Verification items for this drawing (mm, ordinates from the low corner). A direction names the side the tool comes from. Coordinates: 2 decimals unless noted, no trailing zeros. Loops run counter-clockwise (first coordinate to the right, second up) from the corner with the lowest first, then second, coordinate; pieces in that order, holes last. Notation, with made-up numbers: (31, -29) -> (57, -29) arc R15 ccw to (57, -13) -> close; hole circle Ø3 at (47, -5.5). An arc over 180 degrees is marked (long way). Write item = value, one per line.
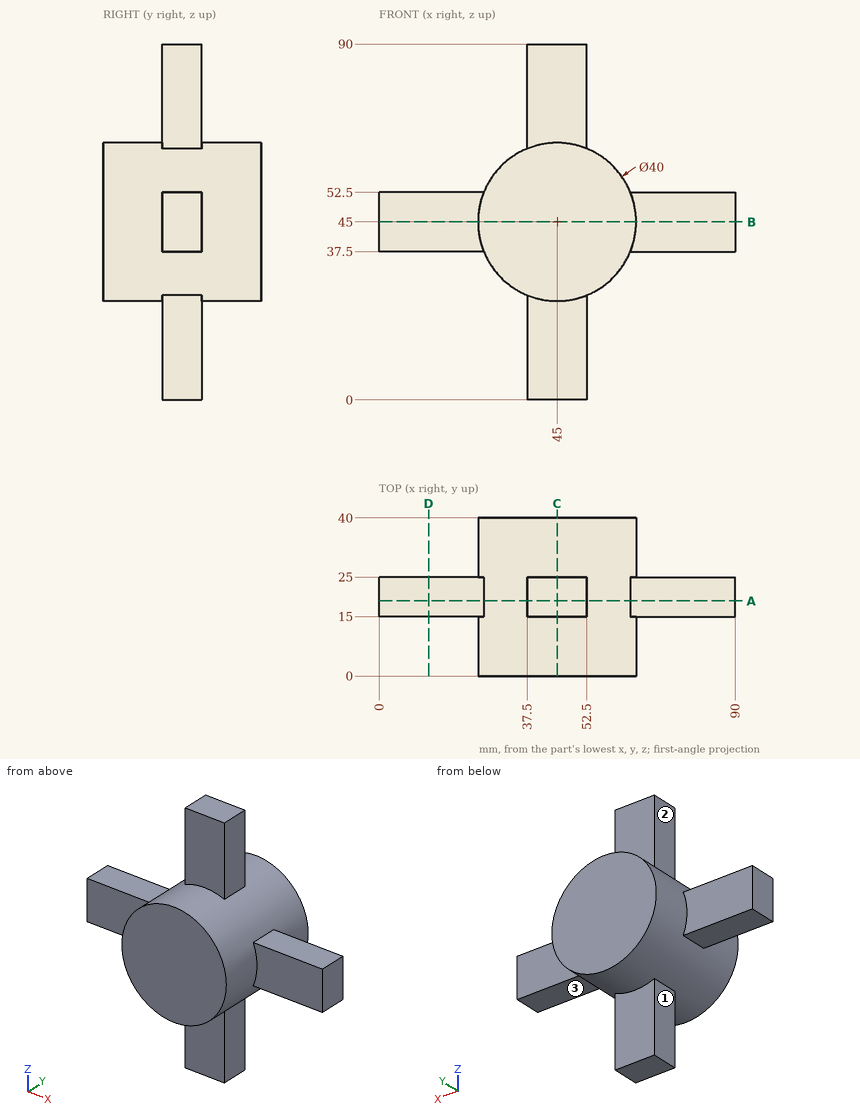
1) Tool access check on the marked faces 1, 2 and 3. Record the directions out of +Z, -Z, +X, -X, +Y, -Y that give a thin tool (end or side, any length) a straight path to the whole face; none if there is none.
Ans:
face_1 = -Z, -X, +Y, -Y
face_2 = +Z, -X, +Y, -Y
face_3 = -Z, +X, +Y, -Y
2) Depth check by flat-ended pin: pin 1 Ø8 at (x, z) = (52, 19) entering from +Y; pin 2 Ø2 at (x, y) = (48, 31.5) entering from -Z; pin 3 Ø11 at (y, z) = (17.5, 73) entering from +X. Enter the tip coordinate at first touch or a pass-through.
Ans:
pin_1 = 25
pin_2 = 25.1
pin_3 = 52.5
3) Sectioned sample at B-B, the plane z = 45. Record the cut outline in (x, y).
Ans:
outline = (0, 15) -> (25, 15) -> (25, 0) -> (65, 0) -> (65, 15) -> (90, 15) -> (90, 25) -> (65, 25) -> (65, 40) -> (25, 40) -> (25, 25) -> (0, 25) -> close
4) Sectioned sample at A-A, the plane y = 19. Record the cut outline in (x, z).
Ans:
outline = (0, 37.5) -> (26.46, 37.5) arc R20 ccw to (37.5, 26.46) -> (37.5, 0) -> (52.5, 0) -> (52.5, 26.46) arc R20 ccw to (63.54, 37.5) -> (90, 37.5) -> (90, 52.5) -> (63.54, 52.5) arc R20 ccw to (52.5, 63.54) -> (52.5, 90) -> (37.5, 90) -> (37.5, 63.54) arc R20 ccw to (26.46, 52.5) -> (0, 52.5) -> close
5) Material ranges on line 1 (X direction, y = 18, z = 73.5); line 2 (Y direction, x = 85.5, z = 43.5), recorded low to high.
Ans:
line_1 = 37.5 to 52.5
line_2 = 15 to 25
6) Sectioned sample at D-D, the plane x = 12.5. Record the cut outline in (y, z), plus the area to 3 significant figures.
Ans:
outline = (15, 37.5) -> (25, 37.5) -> (25, 52.5) -> (15, 52.5) -> close
area = 150 mm2
7) Sectioned sample at C-C, the plane x = 45. Record the cut outline in (y, z).
Ans:
outline = (0, 25) -> (15, 25) -> (15, 0) -> (25, 0) -> (25, 25) -> (40, 25) -> (40, 65) -> (25, 65) -> (25, 90) -> (15, 90) -> (15, 65) -> (0, 65) -> close
